```python
from build123d import *

# Parameters (mm, degrees)
SKETCH1_W           = 35
SKETCH1_H           = 35
BOSS_EXTRUDE1_DEPTH = 30
SKETCH2_W           = 25
SKETCH2_H           = 35
BOSS_EXTRUDE2_DEPTH = 30
SKETCH3_R           = 10
BOSS_EXTRUDE3_DEPTH = 25
BOSS_EXTRUDE4_START = 30
SKETCH4_R           = 10
BOSS_EXTRUDE4_DEPTH = 30
CUT_EXTRUDE1_START  = 10
SKETCH5_R           = 10
SKETCH5_R_2         = 9
CUT_EXTRUDE1_DEPTH  = 10
SKETCH6_W           = 25
SKETCH6_H           = 1
CUT_EXTRUDE2_DEPTH  = 30


with BuildPart() as part:
    # Sketch1 → Boss-Extrude1 (new body)
    with BuildSketch(Plane.XY):
        Rectangle(SKETCH1_W, SKETCH1_H)
    extrude(amount=BOSS_EXTRUDE1_DEPTH)

    # Sketch2 → Boss-Extrude2 (add)
    with BuildSketch(Plane.XY.offset(30)):
        Rectangle(SKETCH2_W, SKETCH2_H)
    extrude(amount=BOSS_EXTRUDE2_DEPTH)

    # Sketch3 → Boss-Extrude3 (add)
    with BuildSketch(Plane.ZY.offset(17.5)):
        with Locations((15, 0)):
            Circle(SKETCH3_R)
    extrude(amount=BOSS_EXTRUDE3_DEPTH)

    # Sketch4 → Boss-Extrude4 (add)
    with BuildSketch(Plane(origin=(17.5, 0, 0), x_dir=(0, 0, -1), z_dir=(1, 0, 0)).offset(BOSS_EXTRUDE4_START)):
        with Locations(Location((-15, 0, 0), (0, 0, 180))):
            Circle(SKETCH4_R)
    extrude(amount=-BOSS_EXTRUDE4_DEPTH)

    # Sketch5 → Cut-Extrude1 (cut)
    with BuildSketch(Plane(origin=(17.5, 0, 0), x_dir=(0, 0, -1), z_dir=(1, 0, 0)).offset(CUT_EXTRUDE1_START)):
        with Locations(Location((-15, 0, 0), (0, 0, 180))):
            Circle(SKETCH5_R)
        with Locations((-15, 0)):
            Circle(SKETCH5_R_2, mode=Mode.SUBTRACT)
    extrude(amount=-CUT_EXTRUDE1_DEPTH, mode=Mode.SUBTRACT)

    # Sketch6 → Cut-Extrude2 (cut)
    with BuildSketch(Plane.XY.offset(60)):
        with Locations((0, 17)):
            Rectangle(SKETCH6_W, SKETCH6_H)
        with Locations((0, -17)):
            Rectangle(SKETCH6_W, SKETCH6_H)
    extrude(amount=-CUT_EXTRUDE2_DEPTH, mode=Mode.SUBTRACT)


solid = part.part
```
Build history of the part. All positions in model axes, mm. A direction names the side the tool comes from. Round coordinates to 2 decimals unless told otherwise and drop trailing zeros. Write each loop counter-clockwise with the first axis right and the second up, starting at its lowest first coordinate (ties: lowest second). Pieces come first, ordered by that corner, then holes.
1) Band-saw the part on D-D, the plane y = 6.5. List the corners of the cut face in (x, z), and give its area (3 significant figures).
2) Band-saw the part on C-C, the plane x = 24.5. List the corners of the cut face in (y, z).
3) Band-saw the part on A-A, the plane z = 15. List the corners of the cut face in (x, y).
4) Band-saw the part on B-B, the plane y = 0. List the corners of the cut face in (x, z), and give its area (3 significant figures).
5) Drill centre lines: probe 1 along X at (y, z) = (-1, 5.5); probe 2 along X at (y, z) = (8, 26.5); probe 3 along X at (y, z) = (-11.5, 39). Where is each one in solid material? Low to high.
6) Mould opens along X. For faces 1 (the flat face through (27.5, -2, 6)), 2 (the flat face through (-17.5, -0.2, 4.8)), 3 (the flat face through (-13, -1, 30)) say: +X half, -X half, draft (parallel to the pull), parting line (faces both ways), or undercut.
7) Pin check, flat tips, straight feed: pin 1 (12 mm diameter, centred on x = 30, y = -12.5, fed in from +Z); pin 2 (1 mm diameter, centred on x = 20, y = 8, fed in from +Z); pin 3 (7.5 mm diameter, centred on x = -6, z = 47.5, fed in from +Y). Stop position of each tip, or through.
8) 3-axis set-ups, long thin cutter, end or side, ignore diameter. For faces 4 (the flat face through (0, 16.5, 45)), 5 (the flat face through (12.5, 0, 45)), 6 (the cylindrical face through (22.57, 2.703, 6.416)): which of +Z, -Z, +X, -X, +Y, -Y reach the whole face in a straight line?
Ans:
1. outline: (-42.5, 7.4) - (-17.5, 7.4) - (-17.5, 0) - (17.5, 0) - (17.5, 8.78) - (27.5, 8.78) - (27.5, 7.4) - (47.5, 7.4) - (47.5, 22.6) - (27.5, 22.6) - (27.5, 21.22) - (17.5, 21.22) - (17.5, 30) - (12.5, 30) - (12.5, 60) - (-12.5, 60) - (-12.5, 30) - (-17.5, 30) - (-17.5, 22.6) - (-42.5, 22.6) - close
1. area: 2,610 mm2
2. outline: circle Ø18 at (0, 15)
3. outline: (-42.5, -10) - (-17.5, -10) - (-17.5, -17.5) - (17.5, -17.5) - (17.5, -9) - (27.5, -9) - (27.5, -10) - (47.5, -10) - (47.5, 10) - (27.5, 10) - (27.5, 9) - (17.5, 9) - (17.5, 17.5) - (-17.5, 17.5) - (-17.5, 10) - (-42.5, 10) - close
4. outline: (-42.5, 5) - (-17.5, 5) - (-17.5, 0) - (17.5, 0) - (17.5, 6) - (27.5, 6) - (27.5, 5) - (47.5, 5) - (47.5, 25) - (27.5, 25) - (27.5, 24) - (17.5, 24) - (17.5, 30) - (12.5, 30) - (12.5, 60) - (-12.5, 60) - (-12.5, 30) - (-17.5, 30) - (-17.5, 25) - (-42.5, 25) - close
4. area: 2,880 mm2
5. probe 1: x = -42.5 to 17.5, 27.5 to 47.5
5. probe 2: x = -17.5 to 17.5
5. probe 3: x = -12.5 to 12.5
6. face 1: undercut
6. face 2: -X half
6. face 3: draft
7. pin 1: stops at z = 22.6
7. pin 2: stops at z = 19.97
7. pin 3: stops at y = 16.5
8. face 4: +Z, +X, -X, +Y
8. face 5: +Z, +X, +Y, -Y
8. face 6: none
